Check sheet for the modelled part. Datum: model origin and axes. Units: mm. Face numbers are marked on the shaded views. A direction names the side the tool comes from. Coordinates: 2 decimals unless noted, no trailing zeros. Write each loop counter-clockwise with the first axis right and the second up, starting at its lowest first coordinate (ties: lowest second). Pieces come first, ordered by that corner, then holes. Notation, with made-up numbers: M 47.5,26.5 L 84.5,26.5 A19 ccw 84.5,59.5 Z; hole C -31.5,13 d3. An arc over 180 degrees is marked long. Answer as CSV lines item,"result". Start each with the question number.
1) Go/stop test with flat-tipped pins: pin 1 Ø8 at (x, z) = (8, 20.5) entering from +Y; pin 2 Ø8 at (x, z) = (27.5, 4) entering from -Y; pin 3 Ø4 at (x, z) = (18, 10) entering from -Y. Record where each tip stops, or that it passes through.
2) Draft check along X on the marked faces 1, 2 and 3. Enter one of: +X half, -X half, draft (parallel to the pull), parting line (faces both ways), or undercut.
3) Section check D-D (z = 19.25). Record the cut outline in (x, y).
4) Section check A-A (z = 14). Record the cut outline in (x, y), and give its area (3 significant figures).
5) Section check C-C (z = 5). Record the cut outline in (x, y), and give its area (3 significant figures).
6) Section check B-B (y = -37.5). Record the cut outline in (x, z), and give its area (3 significant figures).
7) Material ranges on L1, parallel to Y at x = 0, z = 15; L2, parallel to Y at x = -13.5, z = 22.5; L3, parallel to X at y = -2, z = 19.25, recorded low to high. Write a range as [from, to].
8) Access from +Z, -Z, +X, -X, +Y, -Y to the whole of each face (thin tool, end or side, straight path). Record for the marked faces 4 and 5.
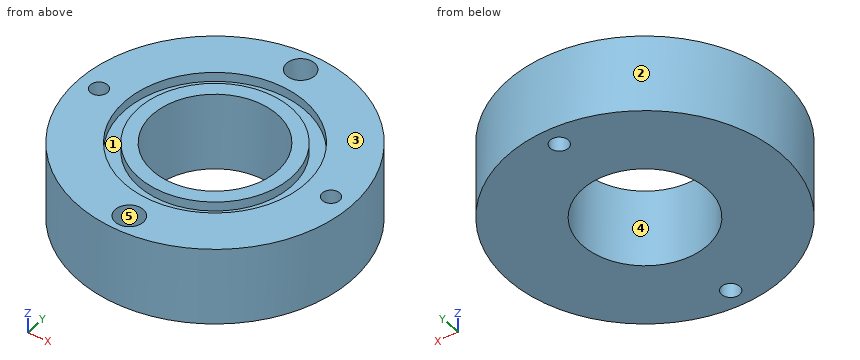
from build123d import *

# Parameters (mm, degrees)
F3_D     = 5.8
F3_DEPTH = 40
F3_TIP   = 1.7424957952
F5_D     = 5.5
F5_DEPTH = 14.4
F5_TIP   = 1.6523667023
F6_R     = 4.5
F6_R_2   = 2.9
F7_DEPTH = 8


with BuildPart() as f1:
    # F0 (on Front) → F1 (revolve)
    with BuildSketch(Plane.XZ):
        Polygon((-20, 0), (-20, 25), (-24.5, 25), (-24.5, 22), (-29, 22), (-29, 25), (-44, 25), (-44, 17), (-44, 8), (-44, 0), align=None)
    revolve(axis=Axis((0, 0, 12.5), (0, 0, -1)))

    # F3
    with Locations(Plane.XY.offset(25)):
        with Locations((0, 37.5), (0, -37.5)):
            Hole(F3_D / 2, depth=F3_DEPTH)
            with Locations((0, 0, -(F3_DEPTH + F3_TIP / 2))):  # 118° drill point
                Cone(0, F3_D / 2, F3_TIP, mode=Mode.SUBTRACT)

    # F5
    with Locations(Plane.XY.offset(25)):
        with Locations((-37.5, 0), (37.5, 0)):
            Hole(F5_D / 2, depth=F5_DEPTH)
            with Locations((0, 0, -(F5_DEPTH + F5_TIP / 2))):  # 118° drill point
                Cone(0, F5_D / 2, F5_TIP, mode=Mode.SUBTRACT)

    # F6 (on face) → F7 (cut)
    with BuildSketch(Plane.XY.offset(25)):
        with Locations((0, 37.5)):
            Circle(F6_R)
        with Locations((0, 37.5)):
            Circle(F6_R_2, mode=Mode.SUBTRACT)
        with Locations((0, -37.5)):
            Circle(F6_R)
        with Locations((0, -37.5)):
            Circle(F6_R_2, mode=Mode.SUBTRACT)
    extrude(amount=-F7_DEPTH, mode=Mode.SUBTRACT)


solid = f1.part
Results found:
1,pin 1,"stops at y = 43.82"
1,pin 2,"stops at y = -37.2"
1,pin 3,"stops at y = -40.99"
2,face 1,"undercut"
2,face 2,"parting line"
2,face 3,"draft"
3,outline,"C 0,0 d88; hole C -37.5,0 d5.5; hole C 0,0 d40; hole C 0,-37.5 d9; hole C 0,37.5 d9; hole C 37.5,0 d5.5"
4,outline,"C 0,0 d88; hole C -37.5,0 d5.5; hole C 0,0 d40; hole C 0,-37.5 d5.8; hole C 0,37.5 d5.8; hole C 37.5,0 d5.5"
4,area,"4,730 mm2"
5,outline,"C 0,0 d88; hole C 0,0 d40; hole C 0,-37.5 d5.8; hole C 0,37.5 d5.8"
5,area,"4,770 mm2"
6,outline,"M -23.02,0 L -2.9,0 L -2.9,17 L -4.5,17 L -4.5,25 L -23.02,25 Z; M 2.9,0 L 23.02,0 L 23.02,25 L 4.5,25 L 4.5,17 L 2.9,17 Z"
6,area,"980 mm2"
7,L1,"y = [-44, -40.4], [-34.6, -20], [20, 34.6], [40.4, 44]"
7,L2,"y = [-41.88, -25.67], [-20.45, -14.76], [14.76, 20.45], [25.67, 41.88]"
7,L3,"x = [-43.95, -39.39], [-35.61, -19.9], [19.9, 35.61], [39.39, 43.95]"
8,face 4,"+Z, -Z"
8,face 5,"+Z"
